The listing builds one solid part. Answer for the finished solid, in the listing's coordinates (mm). A direction names the side the tool comes from. Round coordinates to 2 decimals unless told otherwise and drop trailing zeros. Order: outer loops, then holes, each group sorted by start corner. A loop starts at its lowest first (then second) coordinate and runs counter-clockwise, first axis right, second up. Notation, with made-up numbers: (-29.5, 76) - (8.5, 76) arc R17 cw to (8.5, 82) - close; hole circle Ø7 at (-26, 25). An arc over 180 degrees is marked (long way). Write item = value, one per line.
from build123d import *

# Parameters (mm, degrees)
SKETCH1_R           = 1.7
BOSS_EXTRUDE1_DEPTH = 2
SKETCH2_R           = 1.7
CUT_EXTRUDE1_DEPTH  = 4
SKETCH5_R           = 10
CUT_EXTRUDE2_DEPTH  = 10
SKETCH7_R           = 5
BOSS_EXTRUDE3_DEPTH = 3


with BuildPart() as part:
    # Sketch1 → Boss-Extrude1 (new body)
    with BuildSketch(Plane(origin=(0, 0, 0), x_dir=(1, 0, 0), z_dir=(0, 1, 0))):
        with BuildLine():
            Line((0, 45), (8.125, 45))
            ThreePointArc((8.125, 45), (11.393102806, 46.731897194), (13.125, 50))
            ThreePointArc((13.125, 50), (18.125, 55), (23.125, 50))
            ThreePointArc((23.125, 50), (24.856897194, 46.731897194), (28.125, 45))
            Line((28.125, 45), (116.875, 45))
            ThreePointArc((116.875, 45), (120.143102806, 46.731897194), (121.875, 50))
            ThreePointArc((121.875, 50), (126.875, 55), (131.875, 50))
            ThreePointArc((131.875, 50), (133.606897194, 46.731897194), (136.875, 45))
            Line((136.875, 45), (145, 45))
            ThreePointArc((145, 45), (190, 0), (145, -45))
            Line((145, -45), (136.875, -45))
            ThreePointArc((136.875, -45), (133.606897194, -46.731897194), (131.875, -50))
            ThreePointArc((131.875, -50), (126.875, -55), (121.875, -50))
            ThreePointArc((121.875, -50), (120.143102806, -46.731897194), (116.875, -45))
            Line((116.875, -45), (28.125, -45))
            ThreePointArc((28.125, -45), (24.856897194, -46.731897194), (23.125, -50))
            ThreePointArc((23.125, -50), (18.125, -55), (13.125, -50))
            ThreePointArc((13.125, -50), (11.393102806, -46.731897194), (8.125, -45))
            Line((8.125, -45), (0, -45))
            ThreePointArc((0, -45), (-45, 0), (0, 45))
        make_face()
        with Locations((108.75, -37.5)):
            Circle(SKETCH1_R, mode=Mode.SUBTRACT)
        with Locations((36.25, -37.5)):
            Circle(SKETCH1_R, mode=Mode.SUBTRACT)
        with Locations((36.25, 37.5)):
            Circle(SKETCH1_R, mode=Mode.SUBTRACT)
        with Locations((108.75, 37.5)):
            Circle(SKETCH1_R, mode=Mode.SUBTRACT)
    extrude(amount=BOSS_EXTRUDE1_DEPTH)

    # Sketch2 → Cut-Extrude1 (cut)
    with BuildSketch(Plane(origin=(0, 2, 0), x_dir=(1, 0, 0), z_dir=(0, 1, 0))):
        with Locations((18.11681751, -49.994200378)):
            Circle(SKETCH2_R)
        with Locations((126.86681751, -49.994200378)):
            Circle(SKETCH2_R)
        with Locations((126.86681751, 49.994200378)):
            Circle(SKETCH2_R)
        with Locations((18.11681751, 49.994200378)):
            Circle(SKETCH2_R)
    extrude(amount=-CUT_EXTRUDE1_DEPTH, mode=Mode.SUBTRACT)

    # Sketch5 → Cut-Extrude2 (cut)
    with BuildSketch(Plane(origin=(0, 2, 0), x_dir=(1, 0, 0), z_dir=(0, 1, 0))):
        Circle(SKETCH5_R)
        with Locations((145, 0)):
            Circle(SKETCH5_R)
    extrude(amount=-CUT_EXTRUDE2_DEPTH, mode=Mode.SUBTRACT)

    # Sketch7 → Boss-Extrude3 (add)
    with BuildSketch(Plane(origin=(0, 0, 0), x_dir=(-1, 0, 0), z_dir=(0, -1, 0))):
        with Locations((-72.5, 0)):
            Circle(SKETCH7_R)
    extrude(amount=BOSS_EXTRUDE3_DEPTH)

    # Sketch9 → Cut-Revolve1 (revolve, cut)
    with BuildSketch(Plane.ZY.offset(-72.5)):
        Polygon((0, 0), (0, -3), (-3, -3), align=None)
    revolve(axis=Axis((72.5, 0, 0), (0, -1, 0)), mode=Mode.SUBTRACT)


solid = part.part
Q1. Determine the mould class of faces 1 (the face through (74, 2, -1)), 2 (the face through (133.644, 0.986, 46.695)), 3 (the face through (154.237, 1.014, 3.83)) for opening direction Z: released by +Z, released by -Z, zero draft, split by the parting line, or undercut.
Model answer:
face_1 = zero draft
face_2 = released by +Z
face_3 = undercut
Q2. Section B-B on x = 80 is taken. Determine the outline of the cut face in (y, z).
Model answer:
outline = (0, -45) - (2, -45) - (2, 45) - (0, 45) - close
Q3. Section C-C on z = -31 is taken. Determine the outline of the cut face in (x, y), then the cut area to 3 significant figures.
Model answer:
outline = (-32.62, 0) - (177.62, 0) - (177.62, 2) - (-32.62, 2) - close
area = 420 mm^2
Q4. For faces 4 (the face through (24.82, 0.99, -46.77)), 5 (the face through (67.881, -1.479, 1.915)), 6 (the face through (120.18, 0.99, 46.77)), determine the directions among +Z, -Z, +X, -X, +Y, -Y from which every point of the face is accessible in a straight line to the end or side of a thin tool.
Model answer:
face_4 = -Z, +Y, -Y
face_5 = -Y
face_6 = +Z, +Y, -Y
Q5. Flat-ended cylindrical pins translate along their axes: P1, Ø0.6, axis at x = 4, y = 1, coming from the +Z side; P2, Ø4.5, axis at x = 18.12, z = -49.99, coming from the -Y side; P3, Ø2, axis at y = 1, z = -9, coming from the +X side. Find the tip coordinate at first contact, or state that the pin passes through.
Model answer:
P1 = 45
P2 = 0
P3 = 189.28
Q6. Section A-A on y = 0.8 is taken. Count the separate pieces of the cut face and the enclosed holes in it, then the cut area to 3 significant figures.
Model answer:
separate_pieces = 1
enclosed_holes = 10
area = 19,100 mm^2
Q7. Find the intervals of material crossed by line 1 (X direction, y = 1.3, z = 0); line 2 (Z direction, x = 36.25, y = 1.3); line 3 (X direction, y = 1.7, z = 4), in increasing order. Write a range as from..to.
Model answer:
line_1 = -45..-10, 10..135, 155..190
line_2 = -45..-39.2, -35.8..35.8, 39.2..45
line_3 = -44.82..-9.17, 9.17..135.83, 154.17..189.82
